from build123d import *

# Parameters (mm, degrees)
F3_D            = 6
F3_COPIES_COUNT = 8
F4_SIZE         = 1


# Not quite as in the source:
# - a pattern or mirror of a feature is missing from the dataset's text; its kind, count and spacing are read off the source's solid


with BuildPart() as f1:
    # F0 (on Right) → F1 (revolve)
    with BuildSketch(Plane.YZ):
        Polygon((-6, 0), (0, 0), (0, 39), (-5.7, 39), (-5.7, 31.5), (-12, 31.5), (-12, 15.75), (-6, 15.75), align=None)
    revolve(axis=Axis((0, -15.2627385695, 0), (0, -1, 0)))

    # F3 (through all)
    with Locations(Plane(origin=(0, 0, 0), x_dir=(1, 0, 0), z_dir=(0, 1, 0))):
        with Locations((0, -25)):
            f3 = Hole(F3_D / 2)

    # F3_copies: F3 ×8 about axis
    f3_copies_axis = Axis((0, 0, 0), (0, 1, 0))
    for i in range(1, F3_COPIES_COUNT):
        add(f3.rotate(f3_copies_axis, i * 360 / F3_COPIES_COUNT), mode=Mode.SUBTRACT)

    # F4
    f4_edges = [f1.edges().sort_by_distance(p)[0] for p in [
        (0, -12, -15.75),
        (0, -12, -31.5),
        (0, -5.7, -39),
    ]]
    chamfer(f4_edges, length=F4_SIZE)


solid = f1.part
Part model, mm, in its own coordinate system. A direction names the side the tool comes from. Coordinates: 2 decimals unless noted, no trailing zeros. Loops run counter-clockwise (first coordinate to the right, second up) from the corner with the lowest first, then second, coordinate; pieces in that order, holes last. Notation, with made-up numbers: M -14,-15.75 L 36,-15.75 A29 cw 36,7.25 Z; hole C 57,45.25 d8. An arc over 180 degrees is marked long. Use a Markdown table: item, result. Add a question column.
Q1. Pin check, flat tips, straight feed: P1, Ø1.5, axis at y = -9, z = 16.5, coming from the -X side; P2, Ø16, axis at x = -7, z = 2.5, coming from the -Y side; P3, Ø3, axis at x = -19.5, y = -7, coming from the -Z side. Stop position of each tip, or through.
Q2. Cut at C-C (y = -1). Give the number of separate pieces and of enclosed holes in the cut face, and give its area (3 significant figures).
Q3. Mould opens along X. For faces 1 (the cylindrical face through (-15.3, -6.08, 15.85)), 2 (the flat face through (13, -12, 13)), 3 (the cylindrical face through (-31.232, -8.387, -4.101)) say: +X half, -X half, draft (parallel to the pull), parting line (faces both ways), or undercut.
Q4. Probe L1, parallel to Z at x = 17, y = -6.25; L2, parallel to Y at x = -35, z = 12; L3, parallel to Z at x = -18.5, y = -7.75. List the from-to ranges inside material, lowest first.
Q5. Cut at B-B (z = 0). Write the cut outline in (x, y).
Q6. Cut at A-A (x = 0). Write the cut outline in (y, z), and give its area (4 significant figures).
Q7. Which spindle directions (+Z, -Z, +X, -X, +Y, -Y) get a long thin tool onto all of the face, cutting with end or side? Do faces 4 (the cylindrical face through (-15.616, -8.465, -2.05)), 5 (the cylindrical face through (-26.8, -6.1, 2.4)). Say none if no direction does.
Worked out:
| question | item | result |
|---|---|---|
| 1 | P1 | stops at x = -27.28 |
| 1 | P2 | stops at y = -6 |
| 1 | P3 | stops at z = -33.05 |
| 2 | separate pieces | 1 |
| 2 | enclosed holes | 8 |
| 2 | area | 4,550 mm2 |
| 3 | face 1 | undercut |
| 3 | face 2 | draft |
| 3 | face 3 | parting line |
| 4 | L1 | z = -26.52 to -20.6, -14.76 to 14.76, 20.6 to 26.52 |
| 4 | L2 | y = -5.7 to 0 |
| 4 | L3 | z = -25.5 to -20.56, -14.79 to 14.79, 20.56 to 25.5 |
| 5 | outline | M -39,-4.7 L -38,-5.7 L -31.5,-5.7 L -31.5,-11 L -30.5,-12 L -28,-12 L -28,0 L -39,0 Z; M -22,-12 L -16.75,-12 L -15.75,-11 L -15.75,-6 L 15.75,-6 L 15.75,-11 L 16.75,-12 L 22,-12 L 22,0 L -22,0 Z; M 28,-12 L 30.5,-12 L 31.5,-11 L 31.5,-5.7 L 38,-5.7 L 39,-4.7 L 39,0 L 28,0 Z |
| 6 | outline | M -12,-30.5 L -11,-31.5 L -5.7,-31.5 L -5.7,-38 L -4.7,-39 L 0,-39 L 0,-28 L -12,-28 Z; M -12,-22 L 0,-22 L 0,22 L -12,22 L -12,16.75 L -11,15.75 L -6,15.75 L -6,-15.75 L -11,-15.75 L -12,-16.75 Z; M -12,28 L 0,28 L 0,39 L -4.7,39 L -5.7,38 L -5.7,31.5 L -11,31.5 L -12,30.5 Z |
| 6 | area | 505.5 mm2 |
| 7 | face 4 | -Y |
| 7 | face 5 | +Y, -Y |
